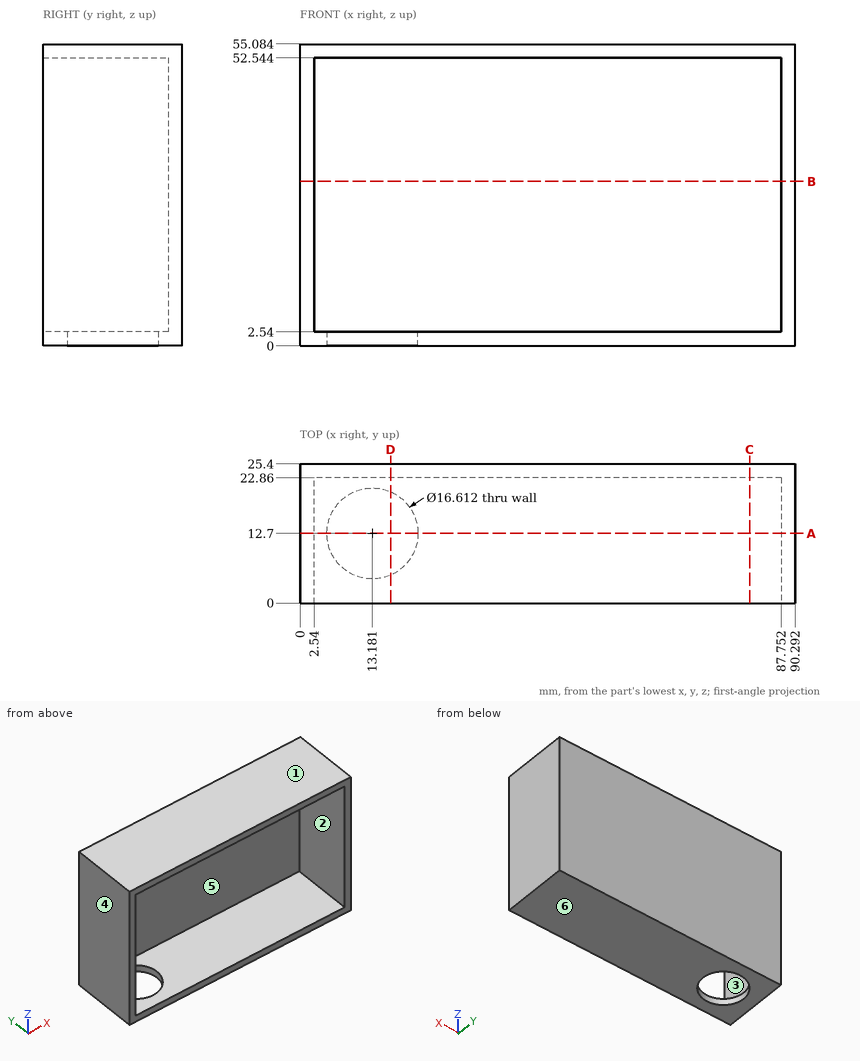
Part print with two shaded views. Sizes in mm from the minimum x, y, z corner. A direction names the side the tool comes from. Coordinates: 2 decimals unless noted, no trailing zeros. Order: outer loops, then holes, each group sorted by start corner. A loop starts at its lowest first (then second) coordinate and runs counter-clockwise, first axis right, second up.
(1) Saw through at D-D, the plane x = 16.5. Write the cut outline in (y, z) (1 decimal).
Solution:
outline: (0, 0) - (5.1, 0) - (5.1, 2.5) - (0, 2.5) - close; (0, 52.5) - (22.9, 52.5) - (22.9, 2.5) - (20.3, 2.5) - (20.3, 0) - (25.4, 0) - (25.4, 55.1) - (0, 55.1) - close
(2) Which spindle directions (+Z, -Z, +X, -X, +Y, -Y) get a long thin tool onto all of the face, cutting with end or side? Do the marked faces 1 and 2. Say none if no direction does.
Solution:
face 1: +Z, +X, -X, +Y, -Y
face 2: -Y
(3) Saw through at C-C, the plane x = 82. Write the cut outline in (y, z), and give its area (3 significant figures).
Solution:
outline: (0, 0) - (25.4, 0) - (25.4, 55.08) - (0, 55.08) - (0, 52.54) - (22.86, 52.54) - (22.86, 2.54) - (0, 2.54) - close
area: 256 mm2
(4) Pin check, flat tip, straight feed: pin 1 Ø6 at (x, z) = (15, 31) entering from -Y. Stop position of the tip, or through.
Solution:
pin 1: stops at y = 22.86
(5) Saw through at B-B, the plane z = 30. Write the cut outline in (x, y).
Solution:
outline: (0, 0) - (2.54, 0) - (2.54, 22.86) - (87.75, 22.86) - (87.75, 0) - (90.29, 0) - (90.29, 25.4) - (0, 25.4) - close
(6) Drill centre lines: L1, parallel to X at y = 12.7, z = 1.75 (1 decimal); L2, parallel to Z at x = 47, y = 14.75; L3, parallel to X at y = 8.5, z = 20. Where is each one in solid material? Low to high.
Solution:
L1: x = 0 to 4.9, 21.5 to 90.3
L2: z = 0 to 2.54, 52.54 to 55.08
L3: x = 0 to 2.54, 87.75 to 90.29
(7) Saw through at A-A, the plane y = 12.7. Write the cut outline in (x, z) (1 decimal).
Solution:
outline: (0, 0) - (4.9, 0) - (4.9, 2.5) - (2.5, 2.5) - (2.5, 52.5) - (87.8, 52.5) - (87.8, 2.5) - (21.5, 2.5) - (21.5, 0) - (90.3, 0) - (90.3, 55.1) - (0, 55.1) - close
(8) Mould opens along X. For the marked faces 3, 4, 5 and 6 say: released by +X, released by -X, zero draft, split by the parting line, or undercut.
Solution:
face 3: undercut
face 4: released by -X
face 5: undercut
face 6: zero draft
